```python
from build123d import *

# Parameters (mm, degrees)
POSICIONAMENTOS_R               = 6.8994
BASE_DEPTH                      = 3
BASE_DENTE_DEPTH                = 3
RAIO_DENTE_R                    = 0.778916794
PADR_OCIRCULAR1_COUNT           = 10
RAIO_DENTE_OF_PADR_OCIRCULAR1_R = 0.778916794
RESSALTO_EXTRUS_O3_DEPTH        = 3
FURO_DE_DI_METRO_3_0_3_1_D      = 3
FURO_DE_DI_METRO_2_6_2_6_1_D    = 2.6
FILETE2_R                       = 5
FILETE3_R                       = 13
FILETE4_R                       = 1


with BuildPart() as part:
    # Posicionamentos → Base (new body)
    with BuildSketch(Plane.XY):
        Circle(POSICIONAMENTOS_R)
    extrude(amount=BASE_DEPTH)

    # Dente → Base Dente (add, through all)
    with BuildSketch(Plane.XY):
        with BuildLine():
            Line((-1.165278514, 8.376570058), (-0.950632674, 6.833594799))
            ThreePointArc((-0.950632674, 6.833594799), (-2.132031851, 6.561719329), (-3.247608255, 6.087262191))
            Line((-3.247608255, 6.087262191), (-3.980894224, 7.461721056))
            ThreePointArc((-3.980894224, 7.461721056), (-4.065642913, 7.734315111), (-4.085914498, 8.019058718))
            ThreePointArc((-4.085914498, 8.019058718), (-4.059577631, 9.094601045), (-3.754624591, 10.126341599))
            ThreePointArc((-3.754624591, 10.126341599), (-3.337383539, 10.271410376), (-2.91455915, 10.399295407))
            ThreePointArc((-2.91455915, 10.399295407), (-2.061405076, 9.743846664), (-1.407910185, 8.889195065))
            ThreePointArc((-1.407910185, 8.889195065), (-1.256942149, 8.64691731), (-1.165278514, 8.376570058))
        make_face()
    base_dente = extrude(amount=BASE_DENTE_DEPTH)

    # Raio Dente
    raio_dente_edges = [part.edges().sort_by_distance(p)[0] for p in [
        (-3.247608255, 6.087262191, 1.5),
        (-0.950632674, 6.833594799, 1.5),
    ]]
    fillet(raio_dente_edges, radius=RAIO_DENTE_R)

    # PadrãoCircular1: Base Dente ×10 about axis, 1 skipped
    padr_ocircular1_axis = Axis((0, 0, 0), (0, 0, -1))
    add([base_dente.rotate(padr_ocircular1_axis, i * 360 / PADR_OCIRCULAR1_COUNT) for i in range(1, PADR_OCIRCULAR1_COUNT) if i not in (8,)])

    # Raio Dente of PadrãoCircular1
    raio_dente_of_padr_ocircular1_edges = [part.edges().sort_by_distance(p)[0] for p in [
        (0.950632674, 6.833594799, 1.5),
        (3.247608255, 6.087262191, 1.5),
        (4.785764232, 4.969726459, 1.5),
        (6.205373212, 3.015802325, 1.5),
        (6.792896515, 1.207591527, 1.5),
        (6.792896515, -1.207591527, 1.5),
        (6.205373212, -3.015802325, 1.5),
        (4.785764232, -4.969726459, 1.5),
        (3.247608255, -6.087262191, 1.5),
        (0.950632674, -6.833594799, 1.5),
        (-0.950632674, -6.833594799, 1.5),
        (-3.247608255, -6.087262191, 1.5),
        (-4.785764232, -4.969726459, 1.5),
        (-6.205373212, -3.015802325, 1.5),
        (-6.205373212, 3.015802325, 1.5),
        (-4.785764232, 4.969726459, 1.5),
    ]]
    fillet(raio_dente_of_padr_ocircular1_edges, radius=RAIO_DENTE_OF_PADR_OCIRCULAR1_R)

    # Braço → Ressalto-extrusão3 (add, through all)
    with BuildSketch(Plane.XY):
        Polygon((0, 4), (-25, 4), (-38, -9), (-25.102702489, -7.416410988), (-21.686291501, -4), (0, -4), align=None)
    extrude(amount=RESSALTO_EXTRUS_O3_DEPTH)

    # Furo de diâmetro Ø3.0 (3)1 (through all)
    with Locations(Plane.XY.offset(3)):
        with Locations((0, 0)):
            Hole(FURO_DE_DI_METRO_3_0_3_1_D / 2)

    # Furo de diâmetro Ø2.6 (2.6)1 (through all)
    with Locations(Plane.XY.offset(3)):
        with Locations((-9, 0)):
            Hole(FURO_DE_DI_METRO_2_6_2_6_1_D / 2)

    # Filete2
    filete2_edges = [part.edges().sort_by_distance(p)[0] for p in [
        (-21.686291501, -4, 1.5),
    ]]
    fillet(filete2_edges, radius=FILETE2_R)

    # Filete3
    filete3_edges = [part.edges().sort_by_distance(p)[0] for p in [
        (-25, 4, 1.5),
    ]]
    fillet(filete3_edges, radius=FILETE3_R)

    # Filete4
    filete4_edges = [part.edges().sort_by_distance(p)[0] for p in [
        (-25.102702489, -7.416410988, 1.5),
        (-38, -9, 1.5),
    ]]
    fillet(filete4_edges, radius=FILETE4_R)


solid = part.part
```
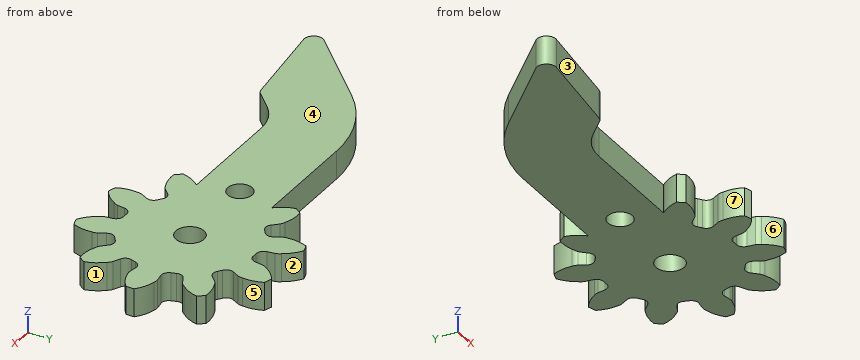
Geometry check sheet. Reference: the model listing, model coordinates, mm. Face numbers are marked on the shaded views. A direction names the side the tool comes from. Round coordinates to 2 decimals unless told otherwise and drop trailing zeros. Write each question's results on one line, items separated by ' | '. Start each with the question number.
Q1. Gauge pin test, flat ends, axial feed: P1, Ø3.5, axis at x = -9, y = 0, coming from the -Z side; P2, Ø0.9, axis at x = -13.5, z = 2, coming from the +Y side; P3, Ø1.5, axis at x = -27.5, z = 2.5, coming from the +Y side. Record the tip position at first contact, or that the pin passes through.
Q2. Release check for a two-part mould opening along X. For the marked faces 4, 5, 6 and 7 record: +X half, -X half, draft (parallel to the pull), parting line (faces both ways), or undercut.
Q3. Access from +Z, -Z, +X, -X, +Y, -Y to the whole of each face (thin tool, end or side, straight path). Record for the marked faces 1, 2 and 3.
Q4. Cross-section at A-A on z = 0.6. State how many separate pieces and enclosed holes the cut face has, and give its area (3 significant figures).
Q5. Thickness scan on line 1 (Y direction, x = 0, z = 0.6); line 2 (X direction, y = 5.5, z = 0.65); line 3 (Y direction, x = 4.5, z = 0.45). Record the ranges inside material, lowest first. Write a range as [from, to].
Answers below:
1) P1: stops at z = 0 | P2: stops at y = 4 | P3: stops at y = 1.87
2) face 4: draft | face 5: +X half | face 6: undercut | face 7: undercut
3) face 1: +Z, -Z, +X | face 2: +Z, -Z, +Y | face 3: +Z, -Z, -Y
4) separate pieces: 1 | enclosed holes: 2 | area: 445 mm²
5) line 1: y = [-6.9, -1.5], [1.5, 6.9] | line 2: x = [-8.85, -5.3], [-4.17, 4.17], [5.3, 8.85] | line 3: y = [-5.3, 5.3]
